Geometry: final body of the model. Coordinates: model frame, mm. A direction names the side the tool comes from. Give positions to 0.01 mm unless a question says otherwise; leave off trailing zeros. Write each loop counter-clockwise with the first axis right and the second up, starting at its lowest first coordinate (ties: lowest second). Pieces come first, ordered by that corner, then holes. Notation, with made-up numbers: (-35, 75) -> (-13, 75) arc R8 ccw to (-13, 88) -> close; hole circle Ø2 at (36, 85). An arc over 180 degrees is marked (long way). Answer as a JSON object with one key per item and string values.
from build123d import *

# Parameters (mm, degrees)
SKETCH1_W           = 25.4
SKETCH1_H           = 25.4
SKETCH1_W_2         = 22.225
SKETCH1_H_2         = 22.225
BOSS_EXTRUDE1_DEPTH = 939.8
SKETCH2_R           = 3.175
CUT_EXTRUDE1_DEPTH  = 26.4
SKETCH3_R           = 3.175
CUT_EXTRUDE2_DEPTH  = 26.4


with BuildPart() as part:
    # Sketch1 → Boss-Extrude1 (new body)
    with BuildSketch(Plane(origin=(0, 0, 0), x_dir=(1, 0, 0), z_dir=(0, 1, 0))):
        Rectangle(SKETCH1_W, SKETCH1_H)
        Rectangle(SKETCH1_W_2, SKETCH1_H_2, mode=Mode.SUBTRACT)
    extrude(amount=BOSS_EXTRUDE1_DEPTH)

    # Sketch2 → Cut-Extrude1 (cut, through all)
    with BuildSketch(Plane(origin=(12.7, 0, 0), x_dir=(0, 0, -1), z_dir=(1, 0, 0))):
        with Locations((0, 12.7)):
            Circle(SKETCH2_R)
        with Locations((0, 927.1)):
            Circle(SKETCH2_R)
    extrude(amount=-CUT_EXTRUDE1_DEPTH, mode=Mode.SUBTRACT)

    # Sketch3 → Cut-Extrude2 (cut, through all)
    with BuildSketch(Plane.XY.offset(12.7)):
        with Locations((0, 12.7)):
            Circle(SKETCH3_R)
        with Locations((0, 927.1)):
            Circle(SKETCH3_R)
    extrude(amount=-CUT_EXTRUDE2_DEPTH, mode=Mode.SUBTRACT)


solid = part.part
Q1. Material intervals for L1, parallel to Z at x = 3.75, y = 497; L2, parallel to Y at x = -12.1, z = 0 (3 decimals), sorted ascending. Write a range as from..to.
Values:
{"L1": "-12.7..-11.11, 11.11..12.7", "L2": "0..9.525, 15.875..923.925, 930.275..939.8"}
Q2. Set-up query: faces 1 (the flat face through (0, 463, 12.7)), 2 (the flat face through (0, 463, 11.112)). Return all of +Z, -Z, +X, -X, +Y, -Y with unobstructed straight access to the full face (end or side cutting, diameter ignored); none if empty.
Values:
{"face 1": "+Z, +X, -X, +Y, -Y", "face 2": "+Y, -Y"}
Q3. First-contact query: P1, Ø4, axis at y = 927.1, z = 0, coming from the +X side. Flat tip, straight axial feed; report the tip coordinate or a pass-through.
Values:
{"P1": "through"}
Q4. Cut plane A-A (y = 722.5). Return the cut outline in (x, z).
Values:
{"outline": "(-12.7, -12.7) -> (12.7, -12.7) -> (12.7, 12.7) -> (-12.7, 12.7) -> close; hole (-11.11, -11.11) -> (11.11, -11.11) -> (11.11, 11.11) -> (-11.11, 11.11) -> close"}
Q5. Mould query, pull axis X, two halves, no side actions, for faces 3 (the flat face through (-12.7, 463, 0)), 4 (the flat face through (-11.3, 939.8, -0.1)), 5 (the flat face through (-11.112, 463, 0)). Classes: pulls with the +X half, pulls with the -X half, needs draft (parallel to the pull), parting line crosses it, or undercut.
Values:
{"face 3": "pulls with the -X half", "face 4": "needs draft", "face 5": "undercut"}
